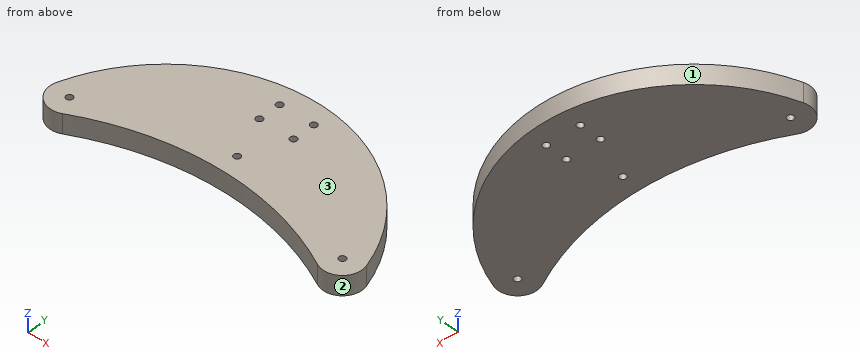
```python
from build123d import *

# Parameters (mm, degrees)
F0_R     = 2.15265
F1_DEPTH = 12.7


with BuildPart() as f1:
    # F0 (on Top) → F1 (new body)
    with BuildSketch(Plane.XY):
        with BuildLine():
            ThreePointArc((18.626667, 4.852237), (101.6, 25.4), (184.573333, 4.852237))
            ThreePointArc((184.573333, 4.852237), (198.667536, 6.359245), (202.587506, 19.980973))
            ThreePointArc((202.587506, 19.980973), (101.6, 93.532141), (0.612494, 19.980973))
            ThreePointArc((0.612494, 19.980973), (4.532464, 6.359245), (18.626667, 4.852237))
        make_face()
        with Locations((12.7, 16.084539)):
            Circle(F0_R, mode=Mode.SUBTRACT)
        with Locations((101.6, 38.1)):
            Circle(F0_R, mode=Mode.SUBTRACT)
        with Locations((190.5, 16.084539)):
            Circle(F0_R, mode=Mode.SUBTRACT)
        with Locations((90.4875, 65.88125)):
            Circle(F0_R, mode=Mode.SUBTRACT)
        with Locations((90.4875, 80.16875)):
            Circle(F0_R, mode=Mode.SUBTRACT)
        with Locations((112.7125, 65.88125)):
            Circle(F0_R, mode=Mode.SUBTRACT)
        with Locations((112.7125, 80.16875)):
            Circle(F0_R, mode=Mode.SUBTRACT)
    extrude(amount=F1_DEPTH)


solid = f1.part
```
Geometry: final body of the model. Coordinates: model frame, mm. Face numbers are marked on the shaded views. Give positions to 0.01 mm unless a question says otherwise; leave off trailing zeros. Write each loop counter-clockwise with the first axis right and the second up, starting at its lowest first coordinate (ties: lowest second). Pieces come first, ordered by that corner, then holes.
1. Section query B-B, the plane y = 38.1. Return loops of the section in (x, z), then the cut area to 3 significant figures.
2. Pin query (flat end, axial travel): P1, Ø3, axis at x = 153, z = 6.5, coming from the +Y side; P2, Ø3, axis at y = 57, z = 6, coming from the +X side; P3, Ø3, axis at x = 153.5, z = 7.5, coming from the -Y side. Return the tip coordinate at first contact, or that it passes through.
3. Draft query along X for the marked faces 1, 2 and 3. Return one class per face: released by +X, released by -X, zero draft, split by the parting line, or undercut.
4. Section query A-A, the plane x = 101.6. Return loops of the section in (y, z), then the cut area to 3 significant figures.
5. Line query: probe 1 along X at (y, z) = (67, 10); probe 2 along Y at (x, z) = (91, 9.25); probe 3 along Y at (x, z) = (190.5, 9). Output: solid intervals per line, ascending.
6. Section query C-C, the plane z = 4.75. Return loops of the section in (x, y).
7. Section query D-D, the plane x = 127. Return loops of the section in (y, z).
Computed:
1. outline: (8.38, 0) - (99.45, 0) - (99.45, 12.7) - (8.38, 12.7) - close; (103.75, 0) - (194.82, 0) - (194.82, 12.7) - (103.75, 12.7) - close
1. area: 2,310 mm2
2. P1: stops at y = 81.07
2. P2: stops at x = 182.99
2. P3: stops at y = 17.19
3. face 1: split by the parting line
3. face 2: undercut
3. face 3: zero draft
4. outline: (25.4, 0) - (35.95, 0) - (35.95, 12.7) - (25.4, 12.7) - close; (40.25, 0) - (93.53, 0) - (93.53, 12.7) - (40.25, 12.7) - close
4. area: 811 mm2
5. probe 1: x = 31.41 to 88.65, 92.33 to 110.87, 114.55 to 171.79
5. probe 2: y = 25.08 to 63.79, 67.97 to 78.08, 82.26 to 93
5. probe 3: y = 3.38 to 13.93, 18.24 to 45.35
6. outline: (0.61, 19.98) arc R12.7 ccw to (18.63, 4.85) arc R177.8 cw to (184.57, 4.85) arc R12.7 ccw to (202.59, 19.98) arc R106.1 ccw to start; hole circle Ø4.31 at (12.7, 16.08); hole circle Ø4.31 at (90.49, 65.88); hole circle Ø4.31 at (90.49, 80.17); hole circle Ø4.31 at (101.6, 38.1); hole circle Ø4.31 at (112.71, 65.88); hole circle Ø4.31 at (112.71, 80.17); hole circle Ø4.31 at (190.5, 16.08)
7. outline: (23.58, 0) - (90.45, 0) - (90.45, 12.7) - (23.58, 12.7) - close
